Autodesk Inventor part; units mm, degrees
ref_plane "YZ Plane" through (0, 0, 0) normal (1, 0, 0) x (0, 1, 0)
ref_plane "XZ Plane" through (0, 0, 0) normal (0, 1, 0) x (-1, 0, 0)
ref_plane "XY Plane" through (0, 0, 0) normal (0, 0, 1) x (1, 0, 0)
sketch "Sketch1" plane through (0, 0, 0) normal (0, 1, 0) x (-1, 0, 0)
  line L0 (0, 0) -> (50.8, 0)
  line L1 (50.8, 0) -> (50.8, -38.1)
  line L2 (50.8, -38.1) -> (0, -38.1)
  line L3 (0, -38.1) -> (0, 0)
  dimension "d0" = 50.8
  dimension "d1" = 38.1
extrude "Extrusion1" add sketch "Sketch1" along normal blind 12.7
fillet "Fillet1" radius 6.35 2 edges at (0, 6.35, 0) (-50.8, 6.35, 0)
sketch "Sketch2" plane through (0, 12.7, 0) normal (0, 1, 0) x (1, 0, 0)
  circle A0 centre (-12.7, 12.7) radius 6.35
  circle A1 centre (-38.1, 12.7) radius 6.35
  line L0 (-50.8, 38.1) -> (-50.8, 6.35)
  line L1 (-44.45, 0) -> (-6.35, 0)
  point P0 (0, 0)
  dimension "d5" = 12.7
  dimension "d6" = 12.7
  dimension "d7" = 12.7
  dimension "d8" = 12.7
extrude "Extrusion2" cut sketch "Sketch2" against normal blind 12.7
sketch "Sketch3" plane through (0, 0, -38.1) normal (0, 0, -1) x (-1, 0, 0)
  line L0 (6.35, 0) -> (0, 0)
  line L1 (0, 0) -> (50.8, 0)
  line L2 (50.8, 0) -> (50.8, 57.15)
  line L3 (50.8, 57.15) -> (0, 57.15)
  line L4 (0, 57.15) -> (0, 0)
  dimension "d11" = 57.15
extrude "Extrusion3" add sketch "Sketch3" along normal blind 12.7
sketch "Sketch4" plane through (0, 0, -38.1) normal (0, 0, 1) x (1, 0, 0)
  line L0 (0, 57.15) -> (0, 12.7)
  line L1 (0, 57.15) -> (-12.7, 57.15)
  line L2 (-12.7, 57.15) -> (-12.7, 12.7)
  line L3 (-12.7, 12.7) -> (0, 12.7)
  line L4 (0, 12.7) -> (0, 57.15)
  line L5 (-50.8, 12.7) -> (-44.45, 12.7)
  line L6 (-50.8, 57.15) -> (0, 57.15)
  line L7 (-50.8, 12.7) -> (-38.1, 12.7)
  line L8 (-38.1, 12.7) -> (-38.1, 57.15)
  line L9 (-38.1, 57.15) -> (-50.8, 57.15)
  line L10 (-50.8, 57.15) -> (-50.8, 12.7)
  point P0 (0, 0)
  dimension "d14" = 12.7
  dimension "d15" = 12.7
sketch "Sketch5" plane through (0, 0, -38.1) normal (0, 0, 1) x (1, 0, 0)
  line L0 (-50.8, 57.15) -> (0, 57.15)
  line L1 (-38.0673, 57.15) -> (-38.0673, 24.8104)
  line L2 (0, 12.7) -> (-50.8, 12.7)
  arc A0 (-50.8, 12.7) -> (-38.0673, 24.8104) centre (-51.1401, 25.8062) ccw
  line L3 (-12.7393, 57.15) -> (-12.7393, 22.9207)
  arc A1 (-12.7393, 22.9207) -> (0, 12.7) centre (0.0454, 25.8063) ccw
  line L4 (-38.0673, 57.15) -> (-50.8, 57.15)
  line L5 (-50.8, 12.7) -> (-50.8, 57.15)
  line L6 (-50.8, 12.7) -> (-50.8, 57.15)
  line L7 (-12.7393, 57.15) -> (0, 57.15)
  line L8 (0, 57.15) -> (0, 12.7)
  line L9 (0, 57.15) -> (0, 12.7)
  point P0 (0, 0)
  dimension "d16" = 13.1064
extrude "Extrusion4" cut sketch "Sketch5" against normal blind 33.3375 contours L0 L1 A0 L5 | L0 L8 A1 L3
sketch "Sketch6" plane through (0, 0, -50.8) normal (0, 0, -1) x (-1, 0, 0)
  line L0 (38.0673, 57.15) -> (12.7393, 57.15)
  circle A0 centre (25.4033, 57.15) radius 12.7
  point P0 (0, 0)
  dimension "d19" = 25.4
extrude "Extrusion5" add sketch "Sketch6" against normal blind 25.4
sketch "Sketch7" plane through (-25.4033, 57.15, -25.4) normal (0, 0, 1) x (1, 0, 0)
  circle A0 centre (0, 0) radius 6.35
  point P0 (25.4033, -57.15)
  dimension "d22" = 12.7
extrude "Extrusion6" cut sketch "Sketch7" against normal blind 2540
Source: CAD feature listing. Evaluate the final solid. Frame: model axes, mm. A direction names the side the tool comes from. Coordinates: 2 decimals unless noted, no trailing zeros. Loops run counter-clockwise (first coordinate to the right, second up) from the corner with the lowest first, then second, coordinate; pieces in that order, holes last. Notation, with made-up numbers: M -34.75,-16.5 L 11.25,-16.5 A33 cw 11.25,20.5 Z; hole C 39,-27.5 d9. An arc over 180 degrees is marked long. Put each result on its own line as item: value. Start each with the question number.
1) Cut plane A-A on z = -12.7. Return the cut outline in (x, y), then the cut area to 3 significant figures.
2) Cut plane D-D on z = -33. Return the cut outline in (x, y), then the cut area to 3 significant figures.
3) Pull-direction query (Z, two-part tool) for faces 1 (the face through (-38.067, 41, -44)), 2 (the face through (-25, 28, -50.8)), 3 (the face through (-1.91, 6.44, -1.81)), 4 (the face through (-34.686, 6.439, -18.054)); classes: pulls with the +Z half, pulls with the -Z half, needs draft (parallel to the pull), parting line crosses it, or undercut.
4) Ray query, L1, parallel to X at y = 7.75, z = -12.7; L2, parallel to X at y = 57, z = -32; L3, parallel to Z at x = -12.7, y = 7. Return the intervals inside material, ascending. Write a range as from..to.
5) Reachability of faces 5 (the face through (-25, 12.7, -19)), 6 (the face through (-23.75, 69.74, -35.46)), 7 (the face through (-26.78, 50.95, -37.92)), 8 (the face through (-19.6, 60.2, -25.4)) from +Z, -Z, +X, -X, +Y, -Y: full face, straight path, thin tool, end or side. Return the list, or none.
6) Cut plane B-B on x = -8. Return the cut outline in (y, z), then the cut area to 3 significant figures.
7) Cut plane C-C on y = 57.15. Return the cut outline in (x, z), then the cut area to 3 significant figures.
8) Contact query for flat-ended pins moving along their axis: pin 1 Ø1 at (x, z) = (-26.5, -39.5) entering from +Y; pin 2 Ø4 at (y, z) = (40.5, -42) entering from -X; pin 3 Ø14.5 at (x, y) = (-25.4, 57.15) entering from +Z. Output: stop coordinate, or through.
The answers:
1. outline: M -50.8,0 L -44.45,0 L -44.45,12.7 L -50.8,12.7 Z; M -31.75,0 L -19.05,0 L -19.05,12.7 L -31.75,12.7 Z; M -6.35,0 L 0,0 L 0,12.7 L -6.35,12.7 Z
1. area: 323 mm²
2. outline: M -50.8,0 L 0,0 L 0,12.7 L -50.8,12.7 Z; C -25.4,57.15 d25.4; hole C -25.4,57.15 d12.7
2. area: 1,030 mm²
3. face 1: needs draft
3. face 2: pulls with the -Z half
3. face 3: pulls with the +Z half
3. face 4: undercut
4. L1: x = -50.8..-44.45, -31.75..-19.05, -6.35..0
4. L2: x = -38.1..-31.75, -19.06..-12.7
4. L3: z = -50.8..-19.05, -6.35..0
5. face 5: +Z, +X, -X
5. face 6: +Z
5. face 7: +Z, -Z
5. face 8: +Z, +X, -X, +Y
6. outline: M 0,-50.8 L 15.46,-50.8 L 15.46,-38.1 L 12.7,-38.1 L 12.7,-16.97 L 0,-16.97 Z; M 0,-8.43 L 12.7,-8.43 L 12.7,0 L 0,0 Z
6. area: 572 mm²
7. outline: M -38.1,-50.8 L -31.75,-50.8 L -31.75,-25.4 L -38.1,-25.4 Z; M -19.05,-50.8 L -12.7,-50.8 L -12.7,-25.4 L -19.05,-25.4 Z
7. area: 323 mm²
8. pin 1: stops at y = 69.84
8. pin 2: stops at x = -38.07
8. pin 3: stops at z = -25.4
